Part model, mm, in its own coordinate system. A direction names the side the tool comes from. Coordinates: 2 decimals unless noted, no trailing zeros. Order: outer loops, then holes, each group sorted by start corner. A loop starts at its lowest first (then second) coordinate and runs counter-clockwise, first axis right, second up. Notation, with made-up numbers: M 61,6 L 89,6 A17 ccw 89,25 Z; hole C -37.75,62 d10. An arc over 180 degrees is marked long. Write item = value, one per line. Start each with the question number.
from build123d import *

# Parameters (mm, degrees)
SKETCH2_W               = 13.25
SKETCH2_H               = 6
CUT_EXTRUDE1_DEPTH      = 17.45
CUT_EXTRUDE1_DEPTH_BACK = 17.45
BOSS_EXTRUDE1_DEPTH     = 1.55
SKETCH4_W               = 12
SKETCH4_H               = 12.75
BOSS_EXTRUDE2_DEPTH     = 8
SKETCH5_W               = 0.5
SKETCH5_H               = 2.85
BOSS_EXTRUDE3_DEPTH     = 8.25


with BuildPart() as part:
    # Sketch1 → Revolve1 (revolve)
    with BuildSketch(Plane.XY):
        with BuildLine():
            Line((16.45, 0), (14.9, 0))
            Line((14.9, 0), (14.9, -12.25))
            Line((14.9, -12.25), (12.5, -12.25))
            Line((12.5, -12.25), (12.5, -6.25))
            Line((12.5, -6.25), (0, -6.25))
            Line((0, -6.25), (0, 6.55))
            ThreePointArc((0, 6.55), (5.638841208, 6.421540892), (11.26598272, 6.0364301))
            ThreePointArc((11.26598272, 6.0364301), (11.913573869, 5.714750188), (12.175, 5.040577629))
            Line((12.175, 5.040577629), (12.175, 3))
            Line((12.175, 3), (13.45, 3))
            ThreePointArc((13.45, 3), (15.571320344, 2.121320344), (16.45, 0))
        make_face()
    revolve(axis=Axis((0, 7.971043953, 0), (0, -1, 0)))

    # Sketch2 → Cut-Extrude1 (cut, two sides)
    with BuildSketch(Plane.XY) as cut_extrude1_sk:
        with Locations((0, -9.25)):
            Rectangle(SKETCH2_W, SKETCH2_H)
    extrude(amount=CUT_EXTRUDE1_DEPTH, mode=Mode.SUBTRACT)
    extrude(cut_extrude1_sk.sketch, amount=-CUT_EXTRUDE1_DEPTH_BACK, mode=Mode.SUBTRACT)

    # Sketch3 → Boss-Extrude1 (add, symmetric)
    with BuildSketch(Plane.XY):
        Polygon((14.9, -10.25), (16.5, -3.25), (15.4, -1.4), (13.9, -1.4), (13.9, -10.25), align=None)
    boss_extrude1 = extrude(amount=BOSS_EXTRUDE1_DEPTH, both=True)

    # Mirror1: Boss-Extrude1 across plane
    add(boss_extrude1.mirror(Plane(origin=(0, 0, 0), x_dir=(0, 0, 1), z_dir=(1, 0, 0))))

    # Sketch4 → Boss-Extrude2 (add)
    with BuildSketch(Plane.XZ.offset(6.25)):
        Rectangle(SKETCH4_W, SKETCH4_H)
    extrude(amount=BOSS_EXTRUDE2_DEPTH)

    # Sketch5 → Boss-Extrude3 (add)
    with BuildSketch(Plane.XZ.offset(14.25)):
        with Locations((2.45, 1.95)):
            Rectangle(SKETCH5_W, SKETCH5_H)
        with Locations((-2.45, -1.95)):
            Rectangle(SKETCH5_W, SKETCH5_H)
    extrude(amount=BOSS_EXTRUDE3_DEPTH)


solid = part.part
Item 1: Cut at B-B, the plane x = 0. Write the cut outline in (y, z) (3 decimals), and give its area (3 significant figures).
Item 2: Flat gauge pins, fed straight in: pin 1 (4 mm diameter, centred on x = 10.5, z = -5.5, fed in from -Y); pin 2 (2 mm diameter, centred on y = -10.5, z = 12, fed in from -X); pin 3 (0.8 mm diameter, centred on y = -8.5, z = 12, fed in from +X). Where does each tip first touch, or does it go through?
Item 3: Wall check: line 1 along X through (y, z) = (-11, -4.5); line 2 along Y through (x, z) = (5, 12.5); line 3 along X through (y, z) = (-14, -4). Give the ranges that are in metal, low to high. Write a range as [from, to].
Item 4: Cut at A-A, the plane y = -11.75. Write the cut outline in (x, z) (3 decimals), and give its area (3 significant figures).
Item 5: Pull direction X, two halves, no side cores. Call faces 1 (the flat face through (-2.7, -18, -2)), 2 (the flat face through (-13, -12.25, -1)), 3 (the flat face through (0, -6.25, -7)), 4 (the cylindrical face through (12.5, -9.2, -0.2)): pulls with the +X half, pulls with the -X half, needs draft (parallel to the pull), parting line crosses it, or undercut.
Item 6: Cut at C-C, the plane y = 4.5. Write the cut outline in (x, z) (3 decimals).
Item 7: 3-axis set-ups, long thin cutter, end or side, ignore diameter. For faces 5 (the flat face through (6, -10, 0)), 6 (the cylindrical face through (-9.66, 4.01, -7.41)), 7 (the flat face through (15.96, -2.34, 0.02)): which of +Z, -Z, +X, -X, +Y, -Y reach the whole face in a straight line?
Filled sheet:
q1.outline = M -14.25,-6.375 L -6.25,-6.375 L -6.25,-14.9 L 0,-14.9 L 0,-16.45 A3 ccw 3,-13.45 L 3,-12.175 L 5.041,-12.175 A1 ccw 6.036,-11.266 A123.826 ccw 6.036,11.266 A1 ccw 5.041,12.175 L 3,12.175 L 3,13.45 A3 ccw 0,16.45 L 0,14.9 L -6.25,14.9 L -6.25,6.375 L -14.25,6.375 Z
q1.area = 464 mm2
q2.pin_1 = -12.25
q2.pin_2 = -10.05
q2.pin_3 = 9.35
q3.line_1 = [-14.2, -11.66], [-6, 6], [11.66, 14.2]
q3.line_2 = [-6.25, 3]
q3.line_3 = [-6, 6]
q4.outline = M -6.625,-13.346 L -6.625,-10.6 A12.5 cw -6.625,10.6 L -6.625,13.346 A14.9 ccw Z; M -6,-6.375 L 6,-6.375 L 6,6.375 L -6,6.375 Z; M 6.625,-13.346 A14.9 ccw 6.625,13.346 L 6.625,10.6 A12.5 cw 6.625,-10.6 Z
q4.area = 293 mm2
q5.face_1 = pulls with the -X half
q5.face_2 = needs draft
q5.face_3 = undercut
q5.face_4 = undercut
q6.outline = C 0,0 d24.35
q7.face_5 = +Z, -Z, -Y
q7.face_6 = +Y
q7.face_7 = +Z, -Z, +X
